For this review, take the finished solid that the model builds, in its own axes (mm). A direction names the side the tool comes from. Round coordinates to 2 decimals unless told otherwise and drop trailing zeros. Order: outer loops, then holes, each group sorted by start corner. A loop starts at its lowest first (then second) coordinate and runs counter-clockwise, first axis right, second up. Notation, with made-up numbers: M -8,50.5 L 2,50.5 A19 cw 2,69.5 Z; hole C -30.75,26.5 d5. An arc over 180 degrees is marked long. Write item = value, one per line. Start each with the question number.
from build123d import *

# Parameters (mm, degrees)
F0_R     = 20
F1_DEPTH = 5
F2_R     = 18
F3_DEPTH = 3
F4_R     = 3.5
F4_R_2   = 1.5
F5_DEPTH = 6
F6_R     = 5
F7_DEPTH = 2


with BuildPart() as f1:
    # F0 (on Top) → F1 (new body)
    with BuildSketch(Plane.XY):
        Circle(F0_R)
    extrude(amount=F1_DEPTH)

    # F2 (on face) → F3 (cut)
    with BuildSketch(Plane.XY.offset(5)):
        Circle(F2_R)
    extrude(amount=-F3_DEPTH, mode=Mode.SUBTRACT)

    # F4 (on face) → F5 (join)
    with BuildSketch(Plane.XY.offset(2)):
        Circle(F4_R)
        Circle(F4_R_2, mode=Mode.SUBTRACT)
    extrude(amount=F5_DEPTH)

    # F6 (on face) → F7 (cut)
    with BuildSketch(Plane(origin=(0, 0, 0), x_dir=(1, 0, 0), z_dir=(0, 0, -1))):
        with Locations((-12.852788, 0)):
            Circle(F6_R)
        with Locations((-8.013582, -10.048714)):
            Circle(F6_R)
        with Locations((2.860014, -12.530542)):
            Circle(F6_R)
        with Locations((11.579962, -5.576616)):
            Circle(F6_R)
        with Locations((11.579962, 5.576616)):
            Circle(F6_R)
        with Locations((2.860014, 12.530542)):
            Circle(F6_R)
        with Locations((-8.013582, 10.048714)):
            Circle(F6_R)
    extrude(amount=-F7_DEPTH, mode=Mode.SUBTRACT)


solid = f1.part
(1) Draft analysis for pull direction X (two halves, no side actions). For faces 1 (the cylindrical face through (-4.336, -19.524, 2.465)), 2 (the flat face through (0, -2, 8)), 3 (the cylindrical face through (-11.98, 13.09, 0.99)), state which applies: released by +X, released by -X, zero draft, split by the parting line, or undercut.
(2) We need section B-B, the plane z = 2.5. Write out the cut boundary in (x, y).
(3) For faces 4 (the flat face through (0, 0, 0)), 5 (the flat face through (0, 0, 2)), list the 3-axis set-ups (+Z, -Z, +X, -X, +Y, -Y) from which the entire face can be reached by the end or side of a thin tool; tool diameter is ignored.
(4) For line 1 along Y through (x, z) = (0, 3.4); line 2 along X through (y, z) = (-14.5, 1.5); line 3 along Z through (x, y) = (-2.5, -6.5), list the stretches that pass through material, from the lowest coordinate up.
(5) Insertion check: pin 1 (8 mm diameter, centred on x = 2.86, y = 12.53, fed in from -Z); pin 2 (4 mm diameter, centred on y = -7.5, z = 6.5, fed in from +X); pin 3 (1.5 mm diameter, centred on y = -3, z = 4.5, fed in from +X); pin 4 (3 mm diameter, centred on y = 11, z = 6, fed in from -X). Each pin has a flat end and moves straight along its axis. Give the tip position at first contact, or say it passes through.
(6) We need section A-A, the plane y = 0. Write out the cut boundary in (x, z), then the cut area to 3 significant figures.
(7) We need section D-D, the plane y = 7. Write out the cut boundary in (x, z) (3 decimals), then the cut area to 3 significant figures.
(8) We need section C-C, the plane x = 9.5. Write out the cut boundary in (y, z).
Values:
q1.face_1 = split by the parting line
q1.face_2 = zero draft
q1.face_3 = undercut
q2.outline = C 0,0 d40; C 0,0 d7; hole C 0,0 d36; hole C 0,0 d3
q3.face_4 = -Z, +X, -X, +Y, -Y
q3.face_5 = +Z
q4.line_1 = -20 to -18, -3.5 to -1.5, 1.5 to 3.5, 18 to 20
q4.line_2 = -13.77 to -10.29, -5.74 to -1.74, 7.46 to 13.77
q4.line_3 = 0 to 2
q5.pin_1 = through
q5.pin_2 = 19.02
q5.pin_3 = 19.87
q5.pin_4 = -17.39
q6.outline = M -20,0 L -17.85,0 L -17.85,2 L -18,2 L -18,5 L -20,5 Z; M -7.85,0 L 20,0 L 20,5 L 18,5 L 18,2 L 3.5,2 L 3.5,8 L 1.5,8 L 1.5,2 L -1.5,2 L -1.5,8 L -3.5,8 L -3.5,2 L -7.85,2 Z
q6.area = 96.0 mm²
q7.outline = M -18.735,0 L -11.977,0 L -11.977,2 L -16.583,2 L -16.583,5 L -18.735,5 Z; M -4.051,0 L 6.787,0 L 6.787,2 L -4.051,2 Z; M 16.373,0 L 18.735,0 L 18.735,5 L 16.583,5 L 16.583,2 L 16.373,2 Z
q7.area = 52.8 mm²
q8.outline = M -17.6,0 L -10.12,0 L -10.12,2 L -15.29,2 L -15.29,5 L -17.6,5 Z; M -1.03,0 L 1.03,0 L 1.03,2 L -1.03,2 Z; M 10.12,0 L 17.6,0 L 17.6,5 L 15.29,5 L 15.29,2 L 10.12,2 Z
